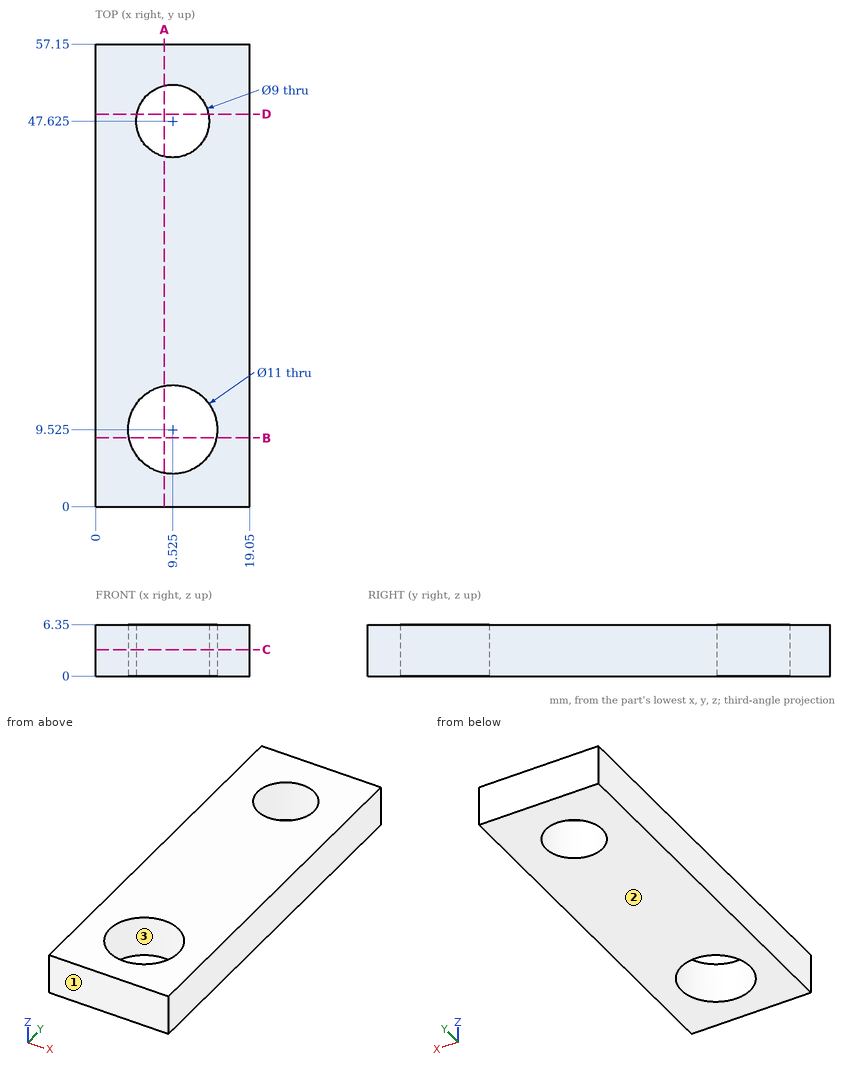
Design review of the part shown in the three views and the two pictorial views. Dimensions are in mm from the part's minimum x, y and z. Give positions to 0.01 mm unless a question says otherwise; leave off trailing zeros. Write each loop counter-clockwise with the first axis right and the second up, starting at its lowest first coordinate (ties: lowest second). Pieces come first, ordered by that corner, then holes.
(1) Add section D-D (y = 48.5). Give the boundary of the cut face in (x, z), and give its area (3 significant figures).
Checked values:
outline: (0, 0) - (5.11, 0) - (5.11, 6.35) - (0, 6.35) - close; (13.94, 0) - (19.05, 0) - (19.05, 6.35) - (13.94, 6.35) - close
area: 64.9 mm2
(2) Add section C-C (z = 3.25). Give the boundary of the cut face in (x, y) (3 decimals), and give its area (3 significant figures).
Checked values:
outline: (0, 0) - (19.05, 0) - (19.05, 57.15) - (0, 57.15) - close; hole circle Ø11 at (9.525, 9.525); hole circle Ø9 at (9.525, 47.625)
area: 930 mm2
(3) Add section B-B (y = 8.5). Give the boundary of the cut face in (x, z).
Checked values:
outline: (0, 0) - (4.12, 0) - (4.12, 6.35) - (0, 6.35) - close; (14.93, 0) - (19.05, 0) - (19.05, 6.35) - (14.93, 6.35) - close
(4) Wall thickness on line 1 along Y through (x, z) = (13.25, 0.75); line 2 along Y through (x, z) = (8.75, 4.25); line 3 along X through (y, z) = (9, 1.5): over which ranges is each line inside the solid? List them lowest first.
Checked values:
line 1: y = 0 to 5.48, 13.57 to 45.1, 50.15 to 57.15
line 2: y = 0 to 4.08, 14.97 to 43.19, 52.06 to 57.15
line 3: x = 0 to 4.05, 15 to 19.05
(5) Add section A-A (x = 8.5). Give the boundary of the cut face in (y, z).
Checked values:
outline: (0, 0) - (4.12, 0) - (4.12, 6.35) - (0, 6.35) - close; (14.93, 0) - (43.24, 0) - (43.24, 6.35) - (14.93, 6.35) - close; (52.01, 0) - (57.15, 0) - (57.15, 6.35) - (52.01, 6.35) - close
(6) Mouldability with a two-part tool opening along Y and no side actions: class the marked faces 1, 2 and 3 as +Y half, -Y half, draft (parallel to the pull), parting line (faces both ways), or undercut.
Checked values:
face 1: -Y half
face 2: draft
face 3: undercut
